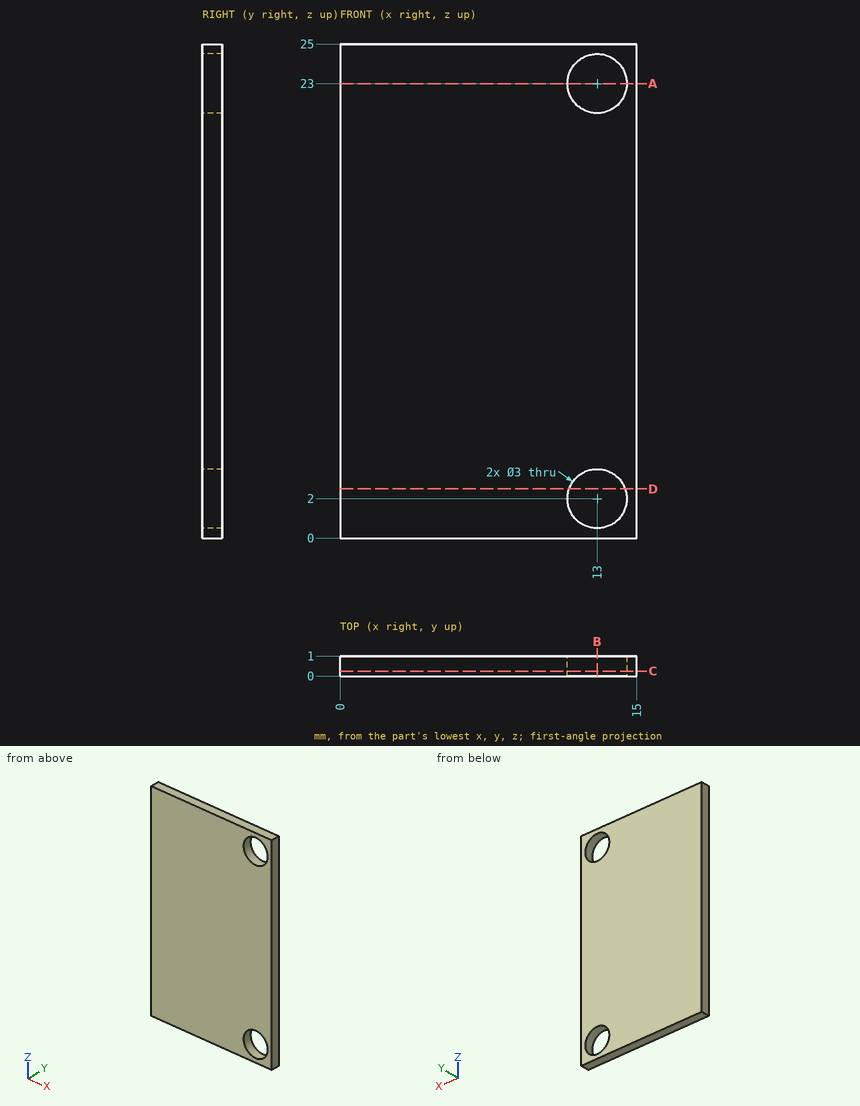
Can you work these out from the drawing? Everything is in mm from the part's minimum corner. Give positions to 0.01 mm unless a question says otherwise; leave off trailing zeros. Loops run counter-clockwise (first coordinate to the right, second up) from the corner with the lowest first, then second, coordinate; pieces in that order, holes last. Notation, with made-up numbers: (-31.75, 53.25) - (24.25, 53.25) arc R31 cw to (24.25, 89.25) - close; hole circle Ø10 at (0, -18.75). An arc over 180 degrees is marked (long way). Use one line per item in the form item = value.
1. I'm going to push a flat-ended pin straight in: pin 1 Ø2.5 at (x, z) = (13, 23) entering from -Y. Where does the tip first touch, or does it pass through?
Response values:
pin_1 = through
2. I want a section at B-B (x = 13). Please give me the cut outline in (y, z).
Response values:
outline = (0, 0) - (1, 0) - (1, 0.5) - (0, 0.5) - close; (0, 3.5) - (1, 3.5) - (1, 21.5) - (0, 21.5) - close; (0, 24.5) - (1, 24.5) - (1, 25) - (0, 25) - close
3. I want a section at D-D (z = 2.5). Please give me the cut outline in (x, y), and give its area (3 significant figures).
Response values:
outline = (0, 0) - (11.59, 0) - (11.59, 1) - (0, 1) - close; (14.41, 0) - (15, 0) - (15, 1) - (14.41, 1) - close
area = 12.2 mm²
4. I want a section at A-A (z = 23). Please give me the cut outline in (x, y), and give its area (3 significant figures).
Response values:
outline = (0, 0) - (11.5, 0) - (11.5, 1) - (0, 1) - close; (14.5, 0) - (15, 0) - (15, 1) - (14.5, 1) - close
area = 12.0 mm²
5. I need wall thicknesses on probe 1 along Z at (x, y) = (13, 0.7); probe 2 along X at (y, z) = (0.6, 23.25); probe 3 along X at (y, z) = (0.7, 21.75). Which ranges of each line are inside material? Lowest first, please.
Response values:
probe_1 = 0 to 0.5, 3.5 to 21.5, 24.5 to 25
probe_2 = 0 to 11.52, 14.48 to 15
probe_3 = 0 to 12.17, 13.83 to 15
6. I want a section at C-C (y = 0.25). Please give me the cut outline in (x, z), and give its area (3 significant figures).
Response values:
outline = (0, 0) - (15, 0) - (15, 25) - (0, 25) - close; hole circle Ø3 at (13, 2); hole circle Ø3 at (13, 23)
area = 361 mm²
